Build history of the part. All positions in model axes, mm. Face numbers are marked on the shaded views. A direction names the side the tool comes from. Round coordinates to 2 decimals unless told otherwise and drop trailing zeros. Write each loop counter-clockwise with the first axis right and the second up, starting at its lowest first coordinate (ties: lowest second). Pieces come first, ordered by that corner, then holes. Notation, with made-up numbers: (-15, -25.5) - (32, -25.5) arc R23 cw to (32, 8.5) - close; hole circle Ø7 at (0.5, 44). An arc over 180 degrees is marked (long way). Answer as a JSON object with one key per item and string values. Group by question number.
Item 1: Slice it at B-B, the plane z = -6.35. List the corners of the cut face in (x, y), then the cut area to 3 significant figures.
Item 2: Probe line 1 (X direction, y = 1.2, z = 38.1); line 2 (Z direction, x = -5.5, y = 10.5); line 3 (Z direction, x = 91.5, y = 1.5). List the from-to ranges inside material, lowest first. Write a range as from..to.
Item 3: Two-plate mould, pull along X, no slides. Class the marked faces 1, 2, 3 and 4: +X half, -X half, draft (parallel to the pull), parting line (faces both ways), or undercut.
Item 4: Slice it at C-C, the plane y = 11.25. List the corners of the cut face in (x, z), then the cut area to 3 significant figures.
Item 5: Slice it at D-D, the plane x = 54. List the corners of the cut face in (y, z), then the cut area to 3 significant figures.
Item 6: Which spindle directions (+Z, -Z, +X, -X, +Y, -Y) get a long thin tool onto all of the face, cutting with end or side? Do the marked faces 5 and 6. Say none if no direction does.
Item 7: Slice it at A-A, the plane z = 38.1. List the corners of the cut face in (x, y).
Item 8: Flat gauge pins, fed straight in: pin 1 (4 mm diameter, centred on x = -30.5, z = 36, fed in from +Y); pin 2 (1 mm diameter, centred on x = 48.5, y = 16.5, fed in from -Z); pin 3 (3.5 mm diameter, centred on y = 2, z = 37, fed in from +X). Where does each tip first touch, or does it go through?
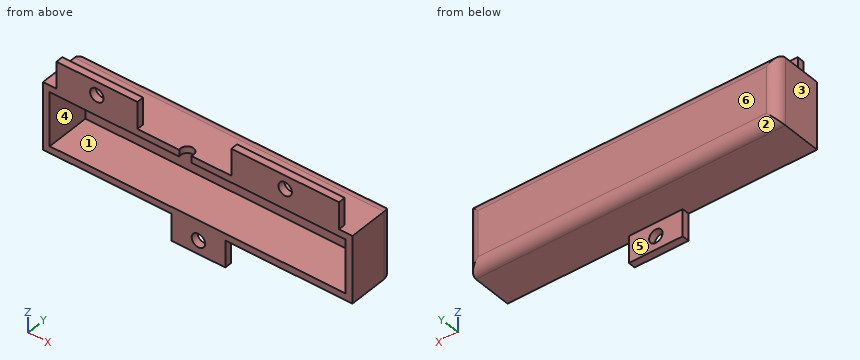
from build123d import *

# Parameters (mm, degrees)
SKETCH1_W           = 146.05
SKETCH1_H           = 23.59
BOSS_EXTRUDE1_DEPTH = 31.75
SKETCH2_W           = 139.69
SKETCH2_H           = 25.39
CUT_EXTRUDE1_DEPTH  = 21
FILLET1_R           = 5
SKETCH3_R           = 3.05
CUT_EXTRUDE2_DEPTH  = 3.18
SKETCH4_W           = 38.19
SKETCH4_H           = 3.39
SKETCH4_W_2         = 50.8
BOSS_EXTRUDE2_DEPTH = 12.7
SKETCH5_W           = 25.4
SKETCH5_H           = 3.39
BOSS_EXTRUDE3_DEPTH = 12.7
SKETCH6_R           = 3.175
CUT_EXTRUDE3_DEPTH  = 12.7
SKETCH7_R           = 3.175
CUT_EXTRUDE4_DEPTH  = 12.7


with BuildPart() as part:
    # Sketch1 → Boss-Extrude1 (new body)
    with BuildSketch(Plane.XY):
        with Locations((25.404065421, 11.795)):
            Rectangle(SKETCH1_W, SKETCH1_H)
    extrude(amount=BOSS_EXTRUDE1_DEPTH)

    # Sketch2 → Cut-Extrude1 (cut)
    with BuildSketch(Plane.XZ):
        with Locations((25.404065421, 15.875)):
            Rectangle(SKETCH2_W, SKETCH2_H)
    extrude(amount=-CUT_EXTRUDE1_DEPTH, mode=Mode.SUBTRACT)

    # Fillet1
    fillet1_edges = [part.edges().sort_by_distance(p)[0] for p in [
        (25.404065421, 23.59, 31.75),
        (25.404065421, 23.59, 0),
        (-47.620934579, 23.59, 15.875),
        (98.429065421, 23.59, 15.875),
    ]]
    fillet(fillet1_edges, radius=FILLET1_R)

    # Sketch3 → Cut-Extrude2 (cut)
    with BuildSketch(Plane.XY.offset(31.75)):
        with Locations((19.559065421, 1.09)):
            Circle(SKETCH3_R)
    extrude(amount=-CUT_EXTRUDE2_DEPTH, mode=Mode.SUBTRACT)

    # Sketch4 → Boss-Extrude2 (add)
    with BuildSketch(Plane.XY.offset(31.75)):
        with Locations((-22.175934579, 1.695)):
            Rectangle(SKETCH4_W, SKETCH4_H)
        with Locations((66.679065421, 1.695)):
            Rectangle(SKETCH4_W_2, SKETCH4_H)
    extrude(amount=BOSS_EXTRUDE2_DEPTH)

    # Sketch5 → Boss-Extrude3 (add)
    with BuildSketch(Plane(origin=(0, 0, 0), x_dir=(-1, 0, 0), z_dir=(0, 0, -1))):
        with Locations((-25.729065421, 1.695)):
            Rectangle(SKETCH5_W, SKETCH5_H)
    extrude(amount=BOSS_EXTRUDE3_DEPTH)

    # Sketch6 → Cut-Extrude3 (cut)
    with BuildSketch(Plane(origin=(0, 3.39, 0), x_dir=(1, 0, 0), z_dir=(0, 1, 0))):
        with Locations((-22.220934579, -38.1)):
            Circle(SKETCH6_R)
        with Locations((66.679065421, -38.1)):
            Circle(SKETCH6_R)
    extrude(amount=-CUT_EXTRUDE3_DEPTH, mode=Mode.SUBTRACT)

    # Sketch7 → Cut-Extrude4 (cut)
    with BuildSketch(Plane(origin=(0, 3.39, 0), x_dir=(1, 0, 0), z_dir=(0, 1, 0))):
        with Locations((25.729065421, 6.35)):
            Circle(SKETCH7_R)
    extrude(amount=-CUT_EXTRUDE4_DEPTH, mode=Mode.SUBTRACT)


solid = part.part
Geometry says:
{
 "1": {"outline": "(13.03, 0) - (22.55, 0) - (22.55, 3.39) - (13.03, 3.39) - close; (28.9, 0) - (38.43, 0) - (38.43, 3.39) - (28.9, 3.39) - close", "area": "64.6 mm^2"},
 "2": {"line 1": "x = -41.27..-25.4, -19.05..-3.08, 41.28..63.5, 69.85..92.08", "line 2": "z = 0..3.18, 28.57..31.75", "line 3": "z = 0..3.18, 28.57..44.45"},
 "3": {"face 1": "undercut", "face 2": "draft", "face 3": "-X half", "face 4": "undercut"},
 "4": {"outline": "(-47.62, 0) - (98.43, 0) - (98.43, 31.75) - (-47.62, 31.75) - close; hole (-44.44, 3.18) - (95.25, 3.18) - (95.25, 28.57) - (-44.44, 28.57) - close", "area": "1,090 mm^2"},
 "5": {"outline": "(0, 0) - (18.59, 0) arc R5 ccw to (23.59, 5) - (23.59, 26.75) arc R5 ccw to (18.59, 31.75) - (3.39, 31.75) - (3.39, 44.45) - (0, 44.45) - (0, 28.57) - (21, 28.57) - (21, 3.18) - (0, 3.18) - close", "area": "248 mm^2"},
 "6": {"face 5": "-Z, +X, -X, +Y", "face 6": "+Z, -Z, +X, -X, +Y"},
 "7": {"outline": "(-41.27, 0) - (-25.4, 0) - (-25.4, 3.39) - (-41.27, 3.39) - close; (-19.05, 0) - (-3.08, 0) - (-3.08, 3.39) - (-19.05, 3.39) - close; (41.28, 0) - (63.5, 0) - (63.5, 3.39) - (41.28, 3.39) - close; (69.85, 0) - (92.08, 0) - (92.08, 3.39) - (69.85, 3.39) - close"},
 "8": {"pin 1": "stops at y = 3.39", "pin 2": "stops at z = 0", "pin 3": "stops at x = 92.08"}
}
